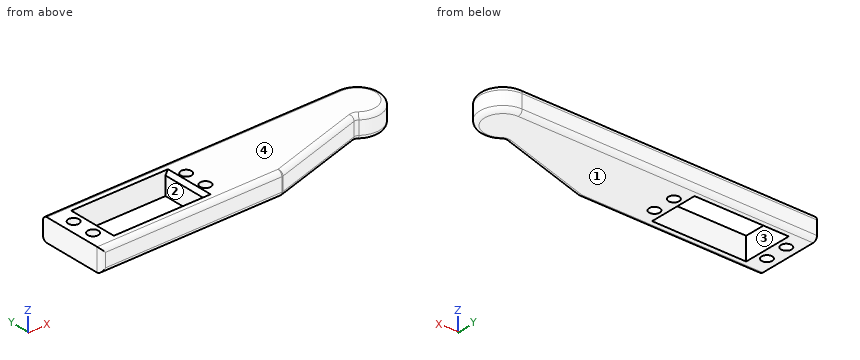
from build123d import *

# Parameters (mm, degrees)
SKETCH1_R           = 2.35
SKETCH1_W           = 41.5
SKETCH1_H           = 22
BOSS_EXTRUDE1_DEPTH = 10
FILLET1_R           = 2
CHAMFER1_SIZE       = 2
CHAMFER1_SIZE2      = 1.154700538


with BuildPart() as part:
    # Sketch1 → Boss-Extrude1 (new body)
    with BuildSketch(Plane.XY):
        with BuildLine():
            Line((-70, 15), (60, 15))
            ThreePointArc((60, 15), (69.302333621, 1.330314836), (53.172672864, -2.306682159))
            Line((53.172672864, -2.306682159), (10, -15))
            Line((10, -15), (-70, -15))
            Line((-70, -15), (-70, 15))
        make_face()
        with Locations((-65, 5)):
            Circle(SKETCH1_R, mode=Mode.SUBTRACT)
        with Locations((-15.4, 5)):
            Circle(SKETCH1_R, mode=Mode.SUBTRACT)
        with Locations(Location((-15.4, -5, 0), (0, 0, 180))):
            Circle(SKETCH1_R, mode=Mode.SUBTRACT)
        with Locations(Location((-65, -5, 0), (0, 0, 180))):
            Circle(SKETCH1_R, mode=Mode.SUBTRACT)
        with Locations((-40.2, 0)):
            Rectangle(SKETCH1_W, SKETCH1_H, mode=Mode.SUBTRACT)
    extrude(amount=BOSS_EXTRUDE1_DEPTH)

    # Fillet1
    fillet1_edges = [part.edges().sort_by_distance(p)[0] for p in [
        (31.586336432, -8.653341079, 10),
        (69.302333621, 1.330314836, 10),
        (-5, 15, 10),
        (-5, 15, 0),
        (69.302333621, 1.330314836, 0),
        (31.586336432, -8.653341079, 0),
        (-30, -15, 0),
        (-30, -15, 10),
        (53.172672864, -2.306682159, 5),
        (10, -15, 5),
        (-70, -15, 5),
    ]]
    fillet(fillet1_edges, radius=FILLET1_R)

    # Chamfer1
    chamfer1_edges = [part.edges().sort_by_distance(p)[0] for p in [
        (-19.45, 0, 10),
    ]]
    chamfer1_side = [part.faces().sort_by_distance(p)[0] for p in [
        (-19.45, 0, 5),
    ]]
    chamfer(chamfer1_edges, length=CHAMFER1_SIZE, length2=CHAMFER1_SIZE2, reference=chamfer1_side[0])


solid = part.part
The listing builds one solid part. Answer for the finished solid, in the listing's coordinates (mm). Face numbers are marked on the shaded views. A direction names the side the tool comes from. Give positions to 0.01 mm unless a question says otherwise; leave off trailing zeros. Write each loop counter-clockwise with the first axis right and the second up, starting at its lowest first coordinate (ties: lowest second). Pieces come first, ordered by that corner, then holes. Notation, with made-up numbers: (36.25, 69) - (62.25, 69) arc R26 cw to (62.25, 83) - close; hole circle Ø6 at (33.5, 61.25). An arc over 180 degrees is marked (long way). One line per question, with ' | ' between items. Start each with the question number.
1. Given P1, Ø1, axis at y = -2.5, z = 1, coming from the +X side; P2, Ø8, axis at x = 34, y = -8, coming from the -Z side; P3, Ø3, axis at y = 0, z = 3, coming from the +X side, each flat-ended and moving along its own axis, determine where each tip first touches the part or whether it passes through.
2. For the marked faces 1 and 2, determine the directions among +Z, -Z, +X, -X, +Y, -Y from which every point of the face is accessible in a straight line to the end or side of a thin tool.
3. Straight lines are drawn through the part: line 1 (Y direction, x = -15.4, z = 5.75); line 2 (Y direction, x = -34, z = 7.5); line 3 (X direction, y = 3.5, z = 7). For each, find the intervals that lie inside material, in ascending order.
4. Section C-C, the plane y = 5 is taken. Count the separate pieces of the cut face and the enclosed holes in it, then the cut area to 3 significant figures.
5. Section A-A, the plane x = -59 is taken. Determine the outline of the cut face in (y, z), then the cut area to 3 significant figures.
6. Determine the mould class of the marked faces 3 and 4 for opening direction Y: +Y half, -Y half, draft (parallel to the pull), parting line (faces both ways), or undercut.
7. Section B-B, the plane z = 3.5 is taken. Determine the outline of the cut face in (x, y), then the cut area to 3 significant figures.
Result:
1) P1: stops at x = 66.87 | P2: stops at z = 0 | P3: stops at x = 69.37
2) face 1: -Z, +X, -X, +Y, -Y | face 2: +Z, -Z
3) line 1: y = -15 to -7.35, -2.65 to 2.65, 7.35 to 15 | line 2: y = -15 to -11, 11 to 15 | line 3: x = -70 to -66.81, -63.19 to -60.95, -19.45 to -17.21, -13.59 to 69.89
4) separate pieces: 4 | enclosed holes: 0 | area: 888 mm2
5) outline: (-15, 2) arc R2 ccw to (-13, 0) - (-11, 0) - (-11, 10) - (-13, 10) arc R2 ccw to (-15, 8) - close; (11, 0) - (13, 0) arc R2 ccw to (15, 2) - (15, 8) arc R2 ccw to (13, 10) - (11, 10) - close | area: 76.6 mm2
6) face 3: undercut | face 4: draft
7) outline: (-70, -13) arc R2 ccw to (-68, -15) - (9.71, -15) arc R2 ccw to (10.28, -14.92) - (52.14, -2.61) arc R2 cw to (53.92, -2.94) arc R10 ccw (long way) to (60, 15) - (-70, 15) - close; hole circle Ø4.7 at (-65, -5); hole circle Ø4.7 at (-65, 5); hole (-60.95, -11) - (-19.45, -11) - (-19.45, 11) - (-60.95, 11) - close; hole circle Ø4.7 at (-15.4, -5); hole circle Ø4.7 at (-15.4, 5) | area: 2,730 mm2
